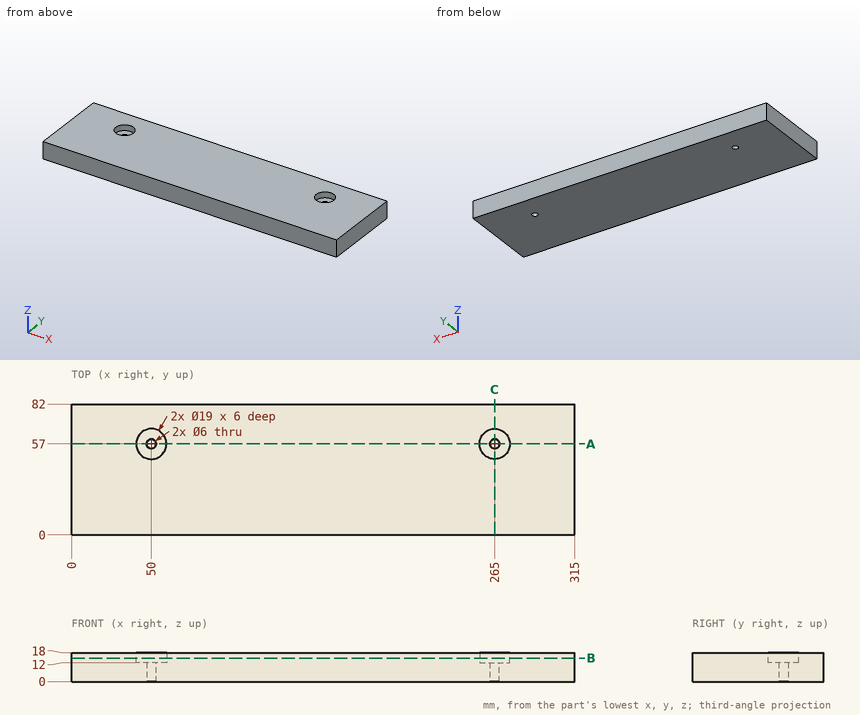
Check sheet for the drawn part. Datum: minimum x, y, z corner. Units: mm. Give positions to 0.01 mm unless a question says otherwise; leave off trailing zeros. Loops run counter-clockwise (first coordinate to the right, second up) from the corner with the lowest first, then second, coordinate; pieces in that order, holes last.
1) Sectioned sample at B-B, the plane z = 14.75. Enter the section's corners in (x, y).
2) Sectioned sample at A-A, the plane y = 57. Enter the section's corners in (x, z).
3) Sectioned sample at C-C, the plane x = 265. Enter the section's corners in (y, z).
4) Thickness scan on line 1 along X through (y, z) = (57, 7.75); line 2 along X through (y, z) = (55.5, 14.25); line 3 along Y through (x, z) = (50, 13.9). Record the ranges inside material, lowest first.
5) Depth check by flat-ended pin: pin 1 Ø5.5 at (x, y) = (265, 57) entering from -Z; pin 2 Ø9.5 at (x, y) = (264, 61.5) entering from +Z. Enter the tip coordinate at first touch or a pass-through.
Answers:
1. outline: (0, 0) - (315, 0) - (315, 82) - (0, 82) - close; hole circle Ø19 at (50, 57); hole circle Ø19 at (265, 57)
2. outline: (0, 0) - (47, 0) - (47, 12) - (40.5, 12) - (40.5, 18) - (0, 18) - close; (53, 0) - (262, 0) - (262, 12) - (255.5, 12) - (255.5, 18) - (59.5, 18) - (59.5, 12) - (53, 12) - close; (268, 0) - (315, 0) - (315, 18) - (274.5, 18) - (274.5, 12) - (268, 12) - close
3. outline: (0, 0) - (54, 0) - (54, 12) - (47.5, 12) - (47.5, 18) - (0, 18) - close; (60, 0) - (82, 0) - (82, 18) - (66.5, 18) - (66.5, 12) - (60, 12) - close
4. line 1: x = 0 to 47, 53 to 262, 268 to 315
4. line 2: x = 0 to 40.62, 59.38 to 255.62, 274.38 to 315
4. line 3: y = 0 to 47.5, 66.5 to 82
5. pin 1: passes through
5. pin 2: stops at z = 12
